```python
from build123d import *

# Parameters (mm, degrees)
SKETCH1_W           = 140
SKETCH1_H           = 70
BOSS_EXTRUDE1_DEPTH = 10
CUT_EXTRUDE1_DEPTH  = 79.89866919
SKETCH3_W           = 10
SKETCH3_H           = 70
CUT_EXTRUDE2_DEPTH  = 10
SKETCH4_W           = 10
SKETCH4_H           = 70
CUT_EXTRUDE3_DEPTH  = 10
SKETCH5_R           = 3.5
CUT_EXTRUDE4_DEPTH  = 71.99166851


with BuildPart() as part:
    # Sketch1 → Boss-Extrude1 (new body)
    with BuildSketch(Plane.XY):
        Rectangle(SKETCH1_W, SKETCH1_H)
    extrude(amount=BOSS_EXTRUDE1_DEPTH)

    # Sketch2 → Cut-Extrude1 (cut, through all)
    with BuildSketch(Plane(origin=(0, 0, 0), x_dir=(-1, 0, 0), z_dir=(0, 0, -1))):
        with BuildLine():
            Line((-44.799329863, 6.296119908), (-37.200670137, 6.296119908))
            ThreePointArc((-37.200670137, 6.296119908), (-37.134647488, 6.307144858), (-37.075789173, 6.339023354))
            ThreePointArc((-37.075789173, 6.339023354), (-34.614722222, 11.376119908), (-37.075789173, 16.413216461))
            ThreePointArc((-37.075789173, 16.413216461), (-37.134647488, 16.445094958), (-37.200670137, 16.456119908))
            Line((-37.200670137, 16.456119908), (-44.799329863, 16.456119908))
            ThreePointArc((-44.799329863, 16.456119908), (-44.865352512, 16.445094958), (-44.924210827, 16.413216461))
            ThreePointArc((-44.924210827, 16.413216461), (-47.385277778, 11.376119908), (-44.924210827, 6.339023354))
            ThreePointArc((-44.924210827, 6.339023354), (-44.865352512, 6.307144858), (-44.799329863, 6.296119908))
        make_face()
        with BuildLine():
            Line((37.200670137, 16.456119908), (44.799329863, 16.456119908))
            ThreePointArc((44.799329863, 16.456119908), (44.865352512, 16.445094958), (44.924210827, 16.413216461))
            ThreePointArc((44.924210827, 16.413216461), (47.385277778, 11.376119908), (44.924210827, 6.339023354))
            ThreePointArc((44.924210827, 6.339023354), (44.865352512, 6.307144858), (44.799329863, 6.296119908))
            Line((44.799329863, 6.296119908), (37.200670137, 6.296119908))
            ThreePointArc((37.200670137, 6.296119908), (37.134647488, 6.307144858), (37.075789173, 6.339023354))
            ThreePointArc((37.075789173, 6.339023354), (34.614722222, 11.376119908), (37.075789173, 16.413216461))
            ThreePointArc((37.075789173, 16.413216461), (37.134647488, 16.445094958), (37.200670137, 16.456119908))
        make_face()
    extrude(amount=-CUT_EXTRUDE1_DEPTH, mode=Mode.SUBTRACT)

    # Sketch3 → Cut-Extrude2 (cut)
    with BuildSketch(Plane(origin=(70, 0, 0), x_dir=(0, 0, -1), z_dir=(1, 0, 0))):
        with Locations((-5, 0)):
            Rectangle(SKETCH3_W, SKETCH3_H)
    extrude(amount=-CUT_EXTRUDE2_DEPTH, mode=Mode.SUBTRACT)

    # Sketch4 → Cut-Extrude3 (cut)
    with BuildSketch(Plane.ZY.offset(70)):
        with Locations((5, 0)):
            Rectangle(SKETCH4_W, SKETCH4_H)
    extrude(amount=-CUT_EXTRUDE3_DEPTH, mode=Mode.SUBTRACT)

    # Sketch5 → Cut-Extrude4 (cut, through all)
    with BuildSketch(Plane(origin=(0, -0.866174302, 12.386869611), x_dir=(1, 0, 0), z_dir=(0, -0.06975647374412544, 0.9975640502598242))):
        with Locations(Location((51, -26.217177022, 0), (0, 0, 270))):
            Circle(SKETCH5_R)
        with Locations(Location((-41, -19.217177022, 0), (0, 0, 270))):
            Circle(SKETCH5_R)
    extrude(amount=-CUT_EXTRUDE4_DEPTH, mode=Mode.SUBTRACT)


solid = part.part
```
Geometry: final body of the model. Coordinates: model frame, mm. A direction names the side the tool comes from. Round coordinates to 2 decimals unless told otherwise and drop trailing zeros. Write each loop counter-clockwise with the first axis right and the second up, starting at its lowest first coordinate (ties: lowest second). Pieces come first, ordered by that corner, then holes. Notation, with made-up numbers: (17.5, 70) -> (24.5, 70) arc R30 cw to (24.5, 101) -> close; hole circle Ø2 at (-5, 12.25). An arc over 180 degrees is marked (long way). Return JSON: item names as keys, results as strings.
Q1. First-contact query: pin 1 Ø12 at (x, y) = (-3.5, -19.5) entering from -Z. Flat tip, straight axial feed; report the tip coordinate or a pass-through.
From the geometry:
{"pin 1": "z = 0"}
Q2. Set-up query: faces 1 (the flat face through (60, 0, 5)), 2 (the cylindrical face through (-34.615, 11.295, 4.93)). Return all of +Z, -Z, +X, -X, +Y, -Y with unobstructed straight access to the full face (end or side cutting, diameter ignored); none if empty.
From the geometry:
{"face 1": "+Z, -Z, +X, +Y, -Y", "face 2": "+Z, -Z"}
Q3. Ray query, line 1 (X direction, y = 7, z = 0.75); line 2 (Y direction, x = 46, z = 6.5); line 3 (Y direction, x = 38.5, z = 5.5). Return the intervals inside material, ascending.
From the geometry:
{"line 1": "-60 to -45.65, -36.35 to 36.35, 45.65 to 60", "line 2": "-35 to 7.4, 15.35 to 35", "line 3": "-35 to 6.3, 16.46 to 35"}
Q4. Section A-A on x = -39. Return the cut outline in (y, z).
From the geometry:
{"outline": "(-35, 0) -> (-22.14, 0) -> (-22.84, 10) -> (-35, 10) -> close; (-17.08, 10) -> (-16.38, 0) -> (6.3, 0) -> (6.3, 10) -> close; (16.46, 0) -> (35, 0) -> (35, 10) -> (16.46, 10) -> close"}
Q5. Mould query, pull axis Y, two halves, no side actions, for faces 3 (the flat face through (-1, 35, 5)), 4 (the flat face through (-1, 0, 0)), 5 (the flat face through (-41, 16.456, 5)). Classes: +Y half, -Y half, draft (parallel to the pull), parting line (faces both ways), or undercut.
From the geometry:
{"face 3": "+Y half", "face 4": "draft", "face 5": "undercut"}
Q6. Section B-B on z = 4.25. Give the number of separate pieces and of enclosed holes in the cut face, and give its area (3 significant figures).
From the geometry:
{"separate pieces": "1", "enclosed holes": "4", "area": "8,090 mm2"}
